from build123d import *

# Parameters (mm, degrees)
BOSS_EXTRUDE1_DEPTH = 23.9141
SKETCH3_OUTSIDE_W   = 26.986
SKETCH3_OUTSIDE_H   = 25.022
SKETCH3_OUTSIDE_R   = 6.35
CUT_EXTRUDE2_DEPTH  = 7.9502
SKETCH4_OUTSIDE_W   = 26.986
SKETCH4_OUTSIDE_H   = 25.022
SKETCH4_OUTSIDE_R   = 6.858
CUT_EXTRUDE3_DEPTH  = 49.801870339
SKETCH5_R           = 2.4892
CUT_EXTRUDE4_DEPTH  = 49.732857286


with BuildPart() as part:
    # Sketch1 → Boss-Extrude1 (new, symmetric)
    with BuildSketch(Plane.XY):
        Polygon((7.332348419, 0), (3.666174209, 6.35), (-3.666174209, 6.35), (-7.332348419, 0), (-3.666174209, -6.35), (3.666174209, -6.35), align=None)
    extrude(amount=BOSS_EXTRUDE1_DEPTH, both=True)

    # Sketch3 outside → Cut-Extrude2 (cut)
    with BuildSketch(Plane.XY.offset(23.9141)):
        Rectangle(SKETCH3_OUTSIDE_W, SKETCH3_OUTSIDE_H)
        Circle(SKETCH3_OUTSIDE_R, mode=Mode.SUBTRACT)
    extrude(amount=-CUT_EXTRUDE2_DEPTH, mode=Mode.SUBTRACT)

    # Sketch4 outside → Cut-Extrude3 (cut, through all)
    with BuildSketch(Plane.XY.offset(23.9141)):
        Rectangle(SKETCH4_OUTSIDE_W, SKETCH4_OUTSIDE_H)
        Circle(SKETCH4_OUTSIDE_R, mode=Mode.SUBTRACT)
    extrude(amount=-CUT_EXTRUDE3_DEPTH, mode=Mode.SUBTRACT)

    # Sketch5 → Cut-Extrude4 (cut, through all)
    with BuildSketch(Plane.XY.offset(23.9141)):
        Circle(SKETCH5_R)
    extrude(amount=-CUT_EXTRUDE4_DEPTH, mode=Mode.SUBTRACT)


solid = part.part
Model file for the job. Use its own axes, mm. A direction names the side the tool comes from. Give positions to 0.01 mm unless a question says otherwise; leave off trailing zeros. Order: outer loops, then holes, each group sorted by start corner. A loop starts at its lowest first (then second) coordinate and runs counter-clockwise, first axis right, second up. Notation, with made-up numbers: (-14.5, 43) - (18.5, 43) arc R34 cw to (18.5, 74) - close; hole circle Ø1 at (1.5, 45.25). An arc over 180 degrees is marked (long way). One line per item, written item: value.
Item 1: Slice it at A-A (y = 0). List the corners of the cut face in (x, z), then the cut area to 3 significant figures.
Response values:
outline: (-6.86, -23.91) - (-2.49, -23.91) - (-2.49, 23.91) - (-6.35, 23.91) - (-6.35, 15.96) - (-6.86, 15.96) - close; (2.49, -23.91) - (6.86, -23.91) - (6.86, 15.96) - (6.35, 15.96) - (6.35, 23.91) - (2.49, 23.91) - close
area: 410 mm2
Item 2: Pin check, flat tips, straight feed: pin 1 Ø3 at (x, y) = (2, -1) entering from -Z; pin 2 Ø2 at (y, z) = (-4.5, -15.5) entering from -X; pin 3 Ø3 at (y, z) = (4, 7) entering from +X; pin 4 Ø3 at (y, z) = (3.5, -14) entering from +X. Stop position of each tip, or through.
Response values:
pin 1: z = -23.91
pin 2: x = -5.31
pin 3: x = 5.89
pin 4: x = 6.18
Item 3: Wall check: line 1 (Y direction, x = 0, z = -12.5); line 2 (Y direction, x = -1, z = 18); line 3 (X direction, y = 6, z = 6.5). Give the ranges that are in metal, low to high.
Response values:
line 1: -6.35 to -2.49, 2.49 to 6.35
line 2: -6.27 to -2.28, 2.28 to 6.27
line 3: -3.32 to 3.32
Item 4: Tool access for faces 1 (the flat face through (3.3, 5.6, 15.964)), 2 (the flat face through (-3.2, -5.7, 15.964)), 3 (the cylindrical face through (-1.38, -6.2, 19.99)), 4 (the flat face through (-3.2, 5.7, 15.964)): list every direction of +Z, -Z, +X, -X, +Y, -Y with a clear straight run to the whole face (end or side of a thin tool).
Response values:
face 1: +Z, +X, +Y
face 2: +Z, -X, -Y
face 3: +Z
face 4: +Z, -X, +Y
Item 5: Slice it at C-C (x = -4.75). List the corners of the cut face in (y, z), then the cut area to 3 significant figures.
Response values:
outline: (-4.47, -23.91) - (4.47, -23.91) - (4.47, 15.96) - (4.21, 15.96) - (4.21, 23.91) - (-4.21, 23.91) - (-4.21, 15.96) - (-4.47, 15.96) - close
area: 424 mm2
Item 6: Slice it at D-D (z = 18). List the corners of the cut face in (x, y).
Response values:
outline: circle Ø12.7 at (0, 0); hole circle Ø4.98 at (0, 0)
Item 7: Slice it at B-B (z = -13). List the corners of the cut face in (x, y).
Response values:
outline: (-6.79, -0.93) - (-4.2, -5.42) arc R6.86 ccw to (-2.59, -6.35) - (2.59, -6.35) arc R6.86 ccw to (4.2, -5.42) - (6.79, -0.93) arc R6.86 ccw to (6.79, 0.93) - (4.2, 5.42) arc R6.86 ccw to (2.59, 6.35) - (-2.59, 6.35) arc R6.86 ccw to (-4.2, 5.42) - (-6.79, 0.93) arc R6.86 ccw to start; hole circle Ø4.98 at (0, 0)
